Autodesk Inventor part; units mm, degrees
ref_plane "YZ Plane" through (0, 0, 0) normal (1, 0, 0) x (0, 1, 0)
ref_plane "XZ Plane" through (0, 0, 0) normal (0, 1, 0) x (-1, 0, 0)
ref_plane "XY Plane" through (0, 0, 0) normal (0, 0, 1) x (1, 0, 0)
sketch "Boceto1" plane through (0, 0, 0) normal (1, 0, 0) x (0, 1, 0)
  line L0 (525, 5.254) -> (525, 25.254)
  line L1 (525, 25.254) -> (540, 25.254)
  arc A0 (540, 25.254) -> (548.4852, 40.5618) centre (540, 35.2596) ccw
  line L2 (548.4852, 40.5618) -> (540.5364, 53.2825)
  line L3 (540.5364, 53.2825) -> (557.4974, 63.8809)
  line L4 (557.4974, 63.8809) -> (565.4462, 51.1602)
  line L5 (525, 15.254) -> (575, 17.0001) construction
  line L6 (549.0169, 58.5817) -> (575, 17.0001) construction
  line L7 (525, 5.254) -> (540, 5.254)
  circle A1 centre (575, 17.0001) radius 5.5
  line L8 (565.4462, 51.1602) -> (571.7687, 41.0421) construction
  line L9 (569.1709, 26.3286) -> (569.5034, 16.8081) construction
  spline S0 degree 4 poles (565.4462, 51.1602) (571.7687, 41.0421) (572.3019, 33) (569.1709, 26.3286) (569.5034, 16.8081) knots 1 1 1 1 1 2 2 2 2 2
  line L10 (580.3797, 18.1518) -> (580.12, 19.0089) construction
  line L11 (580.12, 19.0089) -> (581.7415, 30.4088) construction
  line L12 (581.7415, 30.4088) -> (583, 33.7094) construction
  line L13 (583, 33.7094) -> (588.2679, 31.7007) construction
  line L14 (588.2679, 31.7007) -> (588, 24.7089) construction
  line L15 (588, 24.7089) -> (589.3884, 18.8714) construction
  line L16 (545.515, 5.254) -> (540, 5.254) construction
  line L17 (571.7687, 41.0421) -> (572.3019, 33) construction
  line L18 (572.3019, 33) -> (569.1709, 26.3286) construction
  arc A2 (590.7303, 3.2162) -> (592.5678, 17.3517) centre (589.3333, 10.585) ccw
  arc A3 (568.8646, -8.7498) -> (578.2128, -6.2962) centre (573.2128, -6.2813) ccw
  arc A4 (554.3846, -3.118) -> (559.2353, -5.7559) centre (558.1928, -1.8941) ccw
  spline S1 degree 4 poles (580.3797, 18.1518) (580.12, 19.0089) (581.7415, 30.4088) (583, 33.7094) (588.2679, 31.7007) (588, 24.7089) (589.3884, 18.8714) (592.5678, 17.3517) knots 0 0 0 0 0 1 2 3 4 4 4 4 4
  line L19 (589.3884, 18.8714) -> (592.5678, 17.3517) construction
  spline S2 degree 4 poles (554.3846, -3.118) (552.5025, 2.7386) (550.3005, 4.7218) (545.515, 5.254) (540, 5.254) knots 21.570729 21.570729 21.570729 21.570729 21.570729 22 22 22 22 22
  line L20 (554.3846, -3.118) -> (552.5025, 2.7386) construction
  line L21 (552.5025, 2.7386) -> (550.3005, 4.7218) construction
  line L22 (550.3005, 4.7218) -> (545.515, 5.254) construction
  line L23 (568.8646, -8.7498) -> (566.1112, -3.8997) construction
  line L24 (566.1112, -3.8997) -> (559.2353, -5.7559) construction
  spline S3 degree 2 poles (568.8646, -8.7498) (566.1112, -3.8997) (559.2353, -5.7559) knots 1 1 1 2 2 2
  line L25 (575, 17.0001) -> (525, 17.0001) construction
  line L26 (590.7303, 3.2162) -> (583.3288, 1.8131) construction
  line L27 (583.3288, 1.8131) -> (578.2201, -3.8262) construction
  line L28 (578.2201, -3.8262) -> (578.2128, -6.2962) construction
  spline S4 degree 3 poles (590.7303, 3.2162) (583.3288, 1.8131) (578.2201, -3.8262) (578.2128, -6.2962) knots 1 1 1 1 2 2 2 2
  point P0 (0, 0)
  point P1 (580.3691, 18.1927)
  point P2 (571.0023, 16.8632)
  dimension "d0" = 20
  dimension "d1" = 60
  dimension "d2" = 15
  dimension "d3" = 11
  dimension "d4" = 15
  dimension "d5" = 10
  dimension "d6" = 8
  dimension "d7" = 2
  dimension "d8" = 50
extrude "Extrusión1" add sketch "Boceto1" along normal mid plane 5 contours L0 L1 A0 L2 L3 L4 S0 A1 S1 A2 S4 A3 S3 A4 S2 L7
properties part number "lamina_trasero"
For this review, take the finished solid that the model builds, in its own axes (mm). Round coordinates to 2 decimals unless told otherwise and drop trailing zeros. Write each loop counter-clockwise with the first axis right and the second up, starting at its lowest first coordinate (ties: lowest second). Pieces come first, ordered by that corner, then holes. Notation, with made-up numbers: (87, 33.25) - (142, 33.25) arc R23 cw to (142, 61.25) - close; hole circle Ø7 at (71.5, -23). An arc over 180 degrees is marked (long way). Use a Markdown table: item, result.
Q1. We need section B-B (y = 575). Give the boundary of the cut face in (x, z), plus the area to 3 significant figures.
Derived:
| item | result |
|---|---|
| outline | (-2.5, -10.95) - (2.5, -10.95) - (2.5, 11.5) - (-2.5, 11.5) - close |
| area | 112 mm2 |
Q2. We need section A-A (y = 530.5). Give the boundary of the cut face in (x, z), plus the area to 3 significant figures.
Derived:
| item | result |
|---|---|
| outline | (-2.5, 5.25) - (2.5, 5.25) - (2.5, 25.25) - (-2.5, 25.25) - close |
| area | 100 mm2 |
Q3. The part is to be moulded in two halves that separate along X. For faces 1 (the flat face through (2.5, 560, 18)), 2 (the flat face through (-2.5, 560, 18)), say which applies: pulls with the +X half, pulls with the -X half, needs draft (parallel to the pull), parting line crosses it, or undercut.
Derived:
| item | result |
|---|---|
| face 1 | pulls with the +X half |
| face 2 | pulls with the -X half |
Q4. Clearance check with flat-ended pins moving along their axes: pin 1 (1 mm diameter, centred on x = 1.5, y = 542.5, fed in from +Z); pin 2 (0.8 mm diameter, centred on x = 1, y = 534.5, fed in from -Z); pin 3 (2 mm diameter, centred on x = 0.5, y = 558, fed in from -Z). State where each tip first meets the part, or that it passes through.
Derived:
| item | result |
|---|---|
| pin 1 | stops at z = 54.82 |
| pin 2 | stops at z = 5.25 |
| pin 3 | stops at z = -5.89 |
Q5. Wall thickness on line 1 along Z through (x, y) = (0.7, 535.5); line 2 along Y through (x, z) = (0.75, 15); line 3 along Y through (x, z) = (0.15, 14.5): over which ranges is each line inside the solid? List them lowest first.
Derived:
| item | result |
|---|---|
| line 1 | z = 5.25 to 25.25 |
| line 2 | y = 525 to 569.88, 580.12 to 595.4 |
| line 3 | y = 525 to 570.1, 579.9 to 595.73 |
